Could you check a few things on this drawing? It's one solid part, dimensions in mm from its lowest x, y, z. A direction names the side the tool comes from. Give positions to 0.01 mm unless a question says otherwise; leave off trailing zeros. Loops run counter-clockwise (first coordinate to the right, second up) from the corner with the lowest first, then second, coordinate; pieces in that order, holes last. Notation, with made-up numbers: (79, 66) - (85, 66) arc R36 cw to (85, 102) - close; hole circle Ø9 at (55.25, 31.25). An arc over 180 degrees is marked (long way). Use a Markdown table: item, result.
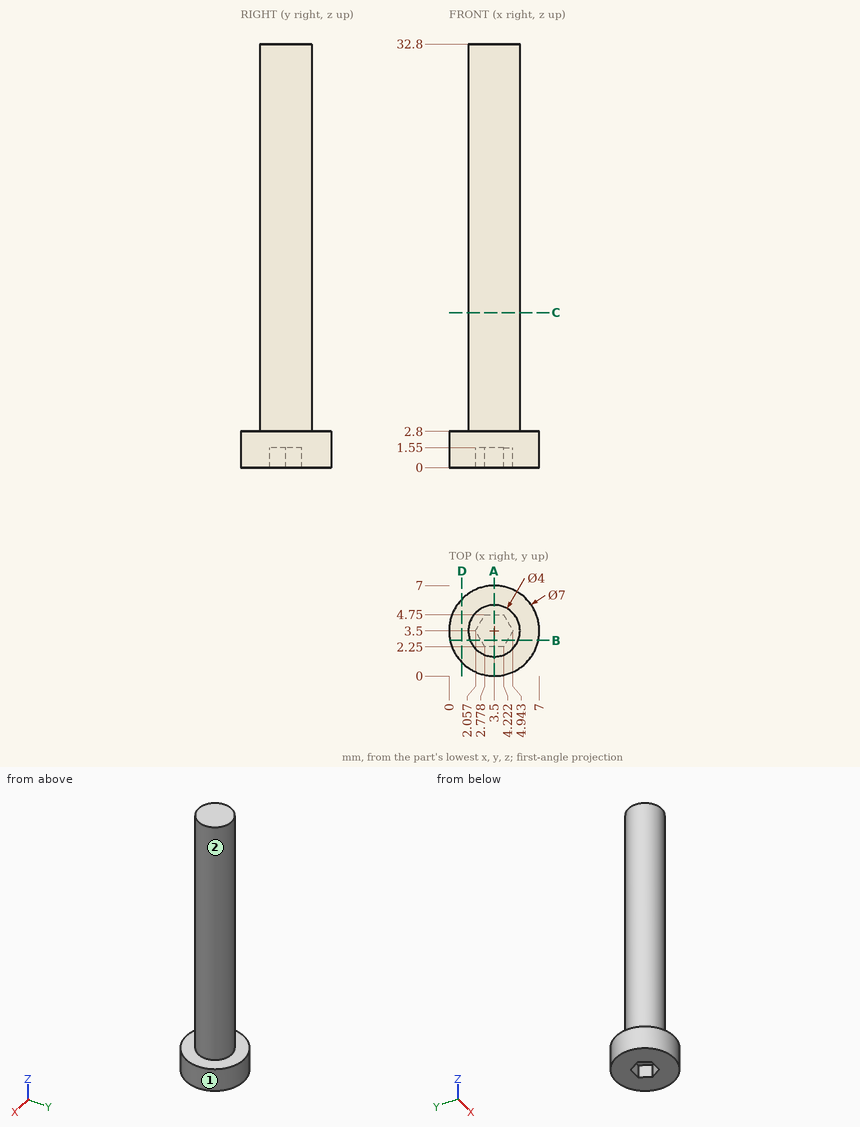
(1) Suppose I cut it at B-B on y = 2.75. Write out the boundary of the cut face in (x, z), plus the area to 3 significant figures.
A:
| item | result |
|---|---|
| outline | (0.08, 0) - (2.49, 0) - (2.49, 1.55) - (4.51, 1.55) - (4.51, 0) - (6.92, 0) - (6.92, 2.8) - (5.35, 2.8) - (5.35, 32.8) - (1.65, 32.8) - (1.65, 2.8) - (0.08, 2.8) - close |
| area | 127 mm2 |
(2) Will these pins go through, and if not, where does the flat tip stop? pin 1 (1 mm diameter, centred on x = 4, z = 25.5, fed in from -Y); pin 2 (2 mm diameter, centred on y = 4, z = 13, fed in from -X); pin 3 (4 mm diameter, centred on y = 6, z = 7.5, fed in from +X).
A:
| item | result |
|---|---|
| pin 1 | y = 1.5 |
| pin 2 | x = 1.5 |
| pin 3 | x = 5.44 |
(3) Suppose I cut it at C-C on z = 12. Write out the boundary of the cut face in (x, y), plus the area to 3 significant figures.
A:
| item | result |
|---|---|
| outline | circle Ø4 at (3.5, 3.5) |
| area | 12.6 mm2 |
(4) Suppose I cut it at A-A on x = 3.5. Write out the boundary of the cut face in (y, z).
A:
| item | result |
|---|---|
| outline | (0, 0) - (2.25, 0) - (2.25, 1.55) - (4.75, 1.55) - (4.75, 0) - (7, 0) - (7, 2.8) - (5.5, 2.8) - (5.5, 32.8) - (1.5, 32.8) - (1.5, 2.8) - (0, 2.8) - close |
(5) If I drill on line 1 (Z direction, x = 5.25, y = 5.75); line 2 (Z direction, x = 3.25, y = 2.75); line 3 (X direction, y = 3.25, z = 10) (1 decimal), over which ranges is the centre line in solid material (lowest first)?
A:
| item | result |
|---|---|
| line 1 | 0 to 2.8 |
| line 2 | 1.55 to 32.8 |
| line 3 | 1.5 to 5.5 |
(6) On a 3-axis mill with a long thin cutter (end or side, diameter ignored), from which of +Z, -Z, +X, -X, +Y, -Y can I reach the whole of each face in a straight line? I mean the marked faces 1 and 2. Say none if no direction works.
A:
| item | result |
|---|---|
| face 1 | +Z, -Z |
| face 2 | +Z |
(7) Suppose I cut it at D-D on x = 1. Write out the boundary of the cut face in (y, z), plus the area to 3 significant figures.
A:
| item | result |
|---|---|
| outline | (1.05, 0) - (5.95, 0) - (5.95, 2.8) - (1.05, 2.8) - close |
| area | 13.7 mm2 |
